```python
from build123d import *

# Parameters (mm, degrees)
SKETCH1_R               = 12.7
BOSS_EXTRUDE1_DEPTH     = 0.2
SKETCH2_R               = 7
BOSS_EXTRUDE2_DEPTH     = 0.8
SKETCH3_R               = 6.2
BOSS_EXTRUDE3_DEPTH     = 5.2
CHAMFER1_SIZE           = 1
SKETCH5_R               = 5
CUT_EXTRUDE1_DEPTH      = 20.000526308
M2_5_TAPPED_HOLE1_D     = 2.05
M2_5_TAPPED_HOLE1_DEPTH = 6.199
M2_5_TAPPED_HOLE1_TIP   = 0.615882135


with BuildPart() as part:
    # Sketch1 → Boss-Extrude1 (new body)
    with BuildSketch(Plane(origin=(0, 0, 0), x_dir=(1, 0, 0), z_dir=(0, 1, 0))):
        with Locations(Location((0, 0, 0), (0, 0, 270))):
            Circle(SKETCH1_R)
    extrude(amount=BOSS_EXTRUDE1_DEPTH)

    # Sketch2 → Boss-Extrude2 (add)
    with BuildSketch(Plane(origin=(0, 0.2, 0), x_dir=(1, 0, 0), z_dir=(0, 1, 0))):
        with Locations(Location((0, 0, 0), (0, 0, 270))):
            Circle(SKETCH2_R)
    extrude(amount=BOSS_EXTRUDE2_DEPTH)

    # Sketch3 → Boss-Extrude3 (add)
    with BuildSketch(Plane(origin=(0, 1, 0), x_dir=(1, 0, 0), z_dir=(0, 1, 0))):
        with Locations(Location((0, 0, 0), (0, 0, 270))):
            Circle(SKETCH3_R)
    extrude(amount=BOSS_EXTRUDE3_DEPTH)

    # Chamfer1
    # the kernel refuses this chamfer: 1 mm, written as the material it takes off along each edge
    with BuildSketch(Plane(origin=(0, 1, 0), x_dir=(0, 0, 1), z_dir=(-1, 0, 0))) as chamfer1_piece_1_section:
        Polygon((7, -CHAMFER1_SIZE), (7 - CHAMFER1_SIZE, 0), (7, 0), align=None)
    chamfer1_piece_1 = revolve(axis=Axis((0, 1, 0), (0, 1, 0)), mode=Mode.PRIVATE)
    chamfer1_piece_1 = split(chamfer1_piece_1, bisect_by=Plane(origin=(0, 0.2, -6.519416157), z_dir=(0, 1, 0)), keep=Keep.TOP, mode=Mode.PRIVATE)
    chamfer1_piece_1 = chamfer1_piece_1 - Plane(origin=(0, 0.519416157, 0), x_dir=(0, 0, 1), z_dir=(0, -1, 0)) * Cylinder(6.2, 28, mode=Mode.PRIVATE)
    add(chamfer1_piece_1, mode=Mode.SUBTRACT)

    # Sketch5 → Cut-Extrude1 (cut, through all)
    with BuildSketch(Plane(origin=(0, 6.2, 0), x_dir=(1, 0, 0), z_dir=(0, 1, 0))):
        with Locations(Location((0, 0, 0), (0, 0, 270))):
            Circle(SKETCH5_R)
    extrude(amount=-CUT_EXTRUDE1_DEPTH, mode=Mode.SUBTRACT)

    # M2.5 Tapped Hole1
    with Locations(Plane(origin=(6.2, 2.7, 0), x_dir=(0, 0, 1), z_dir=(1, 0, 0))):
        with Locations((0, 0)):
            Hole(M2_5_TAPPED_HOLE1_D / 2, depth=M2_5_TAPPED_HOLE1_DEPTH)
            with Locations((0, 0, -(M2_5_TAPPED_HOLE1_DEPTH + M2_5_TAPPED_HOLE1_TIP / 2))):  # 118° drill point
                Cone(0, M2_5_TAPPED_HOLE1_D / 2, M2_5_TAPPED_HOLE1_TIP, mode=Mode.SUBTRACT)


solid = part.part
```
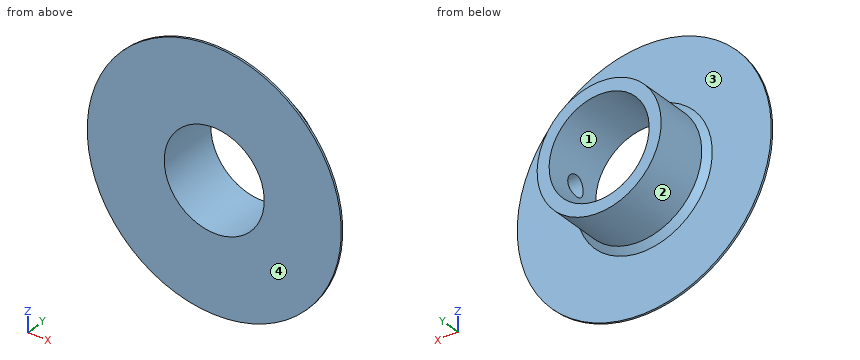
Read the model definition and answer for the solid it produces. Units are mm, in the model's axes. Face numbers are marked on the shaded views. A direction names the side the tool comes from. Round coordinates to 2 decimals unless told otherwise and drop trailing zeros. Write each loop counter-clockwise with the first axis right and the second up, starting at its lowest first coordinate (ties: lowest second). Pieces come first, ordered by that corner, then holes. Notation, with made-up numbers: (15.5, -22.75) -> (69.5, -22.75) arc R26 ccw to (69.5, -1.75) -> close; hole circle Ø11 at (-16.5, -22). An arc over 180 degrees is marked (long way). Answer in a Markdown table with one row per item. Add a question column.
1) Find section D-D, the plane y = 2.7. Determine the outline of the cut face in (x, z) (3 decimals).
2) Consider line 1 (Y direction, x = 5.25, z = 0) (3 decimals); line 2 (X direction, y = 4.5, z = 0); line 3 (X direction, y = 3.5, z = 0). Determine where each line is inside the solid, lowest interval first.
3) Find section A-A, the plane x = 0. Determine the outline of the cut face in (y, z), and give its area (3 significant figures).
4) Given P1, Ø3.5, axis at y = 2.7, z = 0, coming from the +X side; P2, Ø3, axis at x = -9.5, z = 7, coming from the +Y side, each flat-ended and moving along its own axis, determine where each tip first touches the part or whether it passes through.
5) Find section C-C, the plane y = 4.25. Determine the outline of the cut face in (x, z).
6) Determine the mould class of the marked faces 3 and 4 for opening direction Y: pulls with the +Y half, pulls with the -Y half, needs draft (parallel to the pull), parting line crosses it, or undercut.
7) Find section B-B, the plane z = 0. Determine the outline of the cut face in (x, y) (3 decimals).
8) Which of the six approach directions +Z, -Z, +X, -X, +Y, -Y give full straight-line access (tool end or side, diameter ignored) to the marked faces 1 and 2?
Findings below:
| question | item | result |
|---|---|---|
| 1 | outline | (4.894, -1.025) arc R5 cw (long way) to (4.894, 1.025) -> (6.115, 1.025) arc R6.2 ccw (long way) to (6.115, -1.025) -> close |
| 2 | line 1 | 0 to 1.675, 3.725 to 6.2 |
| 2 | line 2 | -6.2 to -5, 5 to 6.2 |
| 2 | line 3 | -6.2 to -5 |
| 3 | outline | (0, -12.7) -> (0.2, -12.7) -> (0.2, -6.8) -> (0.8, -6.2) -> (6.2, -6.2) -> (6.2, -5) -> (0, -5) -> close; (0, 5) -> (6.2, 5) -> (6.2, 6.2) -> (0.8, 6.2) -> (0.2, 6.8) -> (0.2, 12.7) -> (0, 12.7) -> close |
| 3 | area | 17.8 mm² |
| 4 | P1 | x = 6.2 |
| 4 | P2 | y = 0.2 |
| 5 | outline | circle Ø12.4 at (0, 0); hole circle Ø10 at (0, 0) |
| 6 | face 3 | pulls with the +Y half |
| 6 | face 4 | pulls with the -Y half |
| 7 | outline | (-12.7, 0) -> (-5, 0) -> (-5, 6.2) -> (-6.2, 6.2) -> (-6.2, 0.8) -> (-6.8, 0.2) -> (-12.7, 0.2) -> close; (5, 0) -> (12.7, 0) -> (12.7, 0.2) -> (6.8, 0.2) -> (6.2, 0.8) -> (6.2, 1.675) -> (5, 1.675) -> close; (5, 3.725) -> (6.2, 3.725) -> (6.2, 6.2) -> (5, 6.2) -> close |
| 8 | face 1 | +Y, -Y |
| 8 | face 2 | +Y |
